Can you work these out from the model? Positions are in its coordinate system, mm. Face numbers are marked on the shaded views. A direction names the side the tool comes from. Round coordinates to 2 decimals unless told otherwise and drop trailing zeros. Loops run counter-clockwise (first coordinate to the right, second up) from the corner with the lowest first, then second, coordinate; pieces in that order, holes last. Notation, with made-up numbers: (69.25, 78) - (121.25, 78) arc R25 cw to (121.25, 107) - close; hole circle Ø8 at (57, -20.5). An arc over 180 degrees is marked (long way). Answer as CSV lines item,"result".
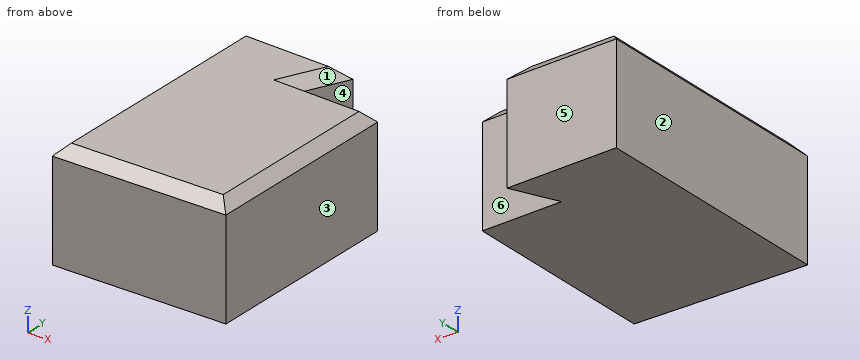
```python
from build123d import *

# Parameters (mm, degrees)
F1_DEPTH = 52.07476
F2_SIZE  = 5.08


with BuildPart() as f1:
    # F0 (on Top) → F1 (new body)
    with BuildSketch(Plane.XY):
        Polygon((-64.110152, 55.120572), (-64.110152, -63.26732), (16.753428, -59.971586), (16.753428, 33.947513), (-21.318547, 33.947513), (-11.569425, 55.120572), align=None)
    extrude(amount=F1_DEPTH)

    # F2
    f2_edges = [f1.edges().sort_by_distance(p)[0] for p in [
        (-23.678362, -61.619453, 52.07476),
        (-64.110152, -4.073374, 52.07476),
        (16.753428, -13.012037, 52.07476),
        (-2.28256, 33.947513, 52.07476),
        (-16.443986, 44.534042, 52.07476),
        (-37.839789, 55.120572, 52.07476),
    ]]
    chamfer(f2_edges, length=F2_SIZE)


solid = f1.part
```
Q1. If I drill on line 1 along Y through (x, z) = (-14, 42.5) (3 decimals); line 2 along Y through (x, z) = (-19, 16); line 3 along X through (y, z) = (44, 8), over which ranges is the centre line in solid material (lowest first)? Write a range as [from, to].
Checks:
line 1,"[-61.225, 33.948], [49.842, 55.121]"
line 2,"[-61.43, 33.95], [38.98, 55.12]"
line 3,"[-64.11, -16.69]"
Q2. Imagine slicing it at A-A (z = 12). Write out the boundary of the cut face in (x, y), then the cut area to 3 significant figures.
Checks:
outline,"(-64.11, -63.27) - (16.75, -59.97) - (16.75, 33.95) - (-21.32, 33.95) - (-11.57, 55.12) - (-64.11, 55.12) - close"
area,"8,740 mm²"
Q3. Imagine slicing it at B-B (x = -3). Write out the boundary of the cut face in (y, z).
Checks:
outline,"(-60.78, 0) - (33.95, 0) - (33.95, 46.99) - (28.87, 52.07) - (-55.69, 52.07) - (-60.78, 46.99) - close"
Q4. We'd pull the mould along Y, two halves only. Please class the marked faces 3, 4, 5 and 6: pulls with the +Y half, pulls with the -Y half, needs draft (parallel to the pull), parting line crosses it, or undercut.
Checks:
face 3,"needs draft"
face 4,"undercut"
face 5,"pulls with the +Y half"
face 6,"undercut"
Q5. On a 3-axis mill with a long thin cutter (end or side, diameter ignored), from which of +Z, -Z, +X, -X, +Y, -Y can I reach the whole of each face in a straight line? I mean the marked faces 1 and 2. Say none if no direction works.
Checks:
face 1,"+Z, +X"
face 2,"+Z, -Z, -X, +Y, -Y"
Q6. I'm going to push flat-ended pins straight in: pin 1 Ø1.5 at (x, z) = (-40.5, 17.5) entering from -Y; pin 2 Ø11.5 at (x, z) = (-1, 26.5) entering from +Y; pin 3 Ø2 at (x, z) = (-33.5, 45) entering from -Y; pin 4 Ø6 at (x, y) = (-45.5, -45.5) entering from -Z. Where does each tip first touch, or does it pass through?
Checks:
pin 1,"y = -62.34"
pin 2,"y = 33.95"
pin 3,"y = -62.06"
pin 4,"z = 0"
